Design review of the part built by this model. Coordinates are the model's own, in mm. A direction names the side the tool comes from. Give positions to 0.01 mm unless a question says otherwise; leave off trailing zeros. Write each loop counter-clockwise with the first axis right and the second up, starting at its lowest first coordinate (ties: lowest second). Pieces come first, ordered by that corner, then holes. Notation, with made-up numbers: M 56,80 L 90,80 A15 cw 90,98 Z; hole C 76.25,-8 d10. An arc over 180 degrees is marked long. One line per item, written item: value. Start each with the question number.
```python
from build123d import *

# Parameters (mm, degrees)
SKETCH_1_W            = 5.5
SKETCH_1_H            = 13
SKETCH_1_W_2          = 7
SKETCH_1_W_3          = 4
SKETCH_1_W_4          = 9
EXTRUDE_1_DEPTH       = 3
HOLE_WIZARD_M31_D     = 3.4
HOLE_WIZARD_M31_DEPTH = 10
HOLE_WIZARD_M31_TIP   = 1.021463052
FILLET_1_R            = 0.5


with BuildPart() as part:
    # Эскиз1 → Бобышка-Вытянуть1 (new body)
    with BuildSketch(Plane(origin=(0, 0, 0), x_dir=(1, 0, 0), z_dir=(0, 1, 0))):
        Polygon((-43.75, -21), (43.75, -21), (43.75, -19.5), (56.25, -19.5), (56.25, -15.5), (59.25, -15.5), (59.25, -5.5), (56.25, -5.5), (56.25, 0), (-56.25, 0), (-56.25, -5.5), (-59.25, -5.5), (-59.25, -15.5), (-56.25, -15.5), (-56.25, -19.5), (-43.75, -19.5), align=None)
        with Locations((-23.625, -9.6)):
            Rectangle(SKETCH_1_W, SKETCH_1_H, mode=Mode.SUBTRACT)
        with Locations((-33.0625, -9.6)):
            Rectangle(SKETCH_1_W, SKETCH_1_H, mode=Mode.SUBTRACT)
        with Locations((-14.1875, -9.6)):
            Rectangle(SKETCH_1_W, SKETCH_1_H, mode=Mode.SUBTRACT)
        with Locations((-4.75, -9.6)):
            Rectangle(SKETCH_1_W, SKETCH_1_H, mode=Mode.SUBTRACT)
        with Locations((16.375, -9.6)):
            Rectangle(SKETCH_1_W_2, SKETCH_1_H, mode=Mode.SUBTRACT)
        with Locations((5.4375, -9.6)):
            Rectangle(SKETCH_1_W_2, SKETCH_1_H, mode=Mode.SUBTRACT)
        with Locations((27.3125, -9.6)):
            Rectangle(SKETCH_1_W_2, SKETCH_1_H, mode=Mode.SUBTRACT)
        with Locations((-41.75, -9.6)):
            Rectangle(SKETCH_1_W_3, SKETCH_1_H, mode=Mode.SUBTRACT)
        with Locations((39.25, -9.6)):
            Rectangle(SKETCH_1_W_4, SKETCH_1_H, mode=Mode.SUBTRACT)
    extrude(amount=EXTRUDE_1_DEPTH)

    # Отверстие с зазором M31
    with Locations(Plane(origin=(0, 3, 0), x_dir=(1, 0, 0), z_dir=(0, 1, 0))):
        with Locations((50, -9.6), (-50, -9.6)):
            Hole(HOLE_WIZARD_M31_D / 2, depth=HOLE_WIZARD_M31_DEPTH)
            with Locations((0, 0, -(HOLE_WIZARD_M31_DEPTH + HOLE_WIZARD_M31_TIP / 2))):  # 118° drill point
                Cone(0, HOLE_WIZARD_M31_D / 2, HOLE_WIZARD_M31_TIP, mode=Mode.SUBTRACT)

    # Скругление1
    fillet_1_edges = [part.edges().sort_by_distance(p)[0] for p in [
        (-56.25, 1.5, 19.5),
        (-59.25, 1.5, 15.5),
        (-59.25, 1.5, 5.5),
        (-56.25, 1.5, 0),
        (56.25, 1.5, 0),
        (59.25, 1.5, 5.5),
        (59.25, 1.5, 15.5),
        (56.25, 1.5, 19.5),
    ]]
    fillet(fillet_1_edges, radius=FILLET_1_R)


solid = part.part
```
Q1. Take a section at C-C, the plane y = 2.3. State how many separate pieces and enclosed holes the cut face has, then the cut area to 3 significant figures.
Q2. Machinability: for faces 4 (the face through (-50, 1, 19.5)), 5 (the face through (-11.438, 1, 10)), which of the approach directions +Z, -Z, +X, -X, +Y, -Y give a long, thin tool a straight path to every point of the face, cutting with its end or side? Answer none if there is none.
Q3. The part is to be moulded in two halves that separate along Z. For faces 1 (the face through (-56.25, 1, 17)), 2 (the face through (34.75, 1, 10)), 3 (the face through (50, 1, 19.5)), say which applies: pulls with the +Z half, pulls with the -Z half, needs draft (parallel to the pull), parting line crosses it, or undercut.
Q4. Take a section at D-D, the plane z = 17.5. Give the boundary of the cut face in (x, y), then the cut area to 4 significant figures.
Q5. Take a section at B-B, the plane x = -50. Give the boundary of the cut face in (y, z), then the cut area to 3 significant figures.
Q6. Take a section at A-A, the plane x = 29.5. Give the boundary of the cut face in (y, z).
Q7. Wall thickness on line 1 (Z direction, x = -33, y = 0.75); line 2 (Z direction, x = 50, y = 1.1); line 3 (X direction, y = 0.1, z = 1.5): over which ranges is each line inside the solid? List them lowest first. Write a range as from..to.
Q8. For P1, Ø1.2, axis at x = -58, y = 1, coming from the -Z side; P2, Ø5, axis at x = 30.5, z = 9, coming from the -Y side; P3, Ø1.6, axis at y = 2, z = 20, coming from the -X side, all flat-tipped, find the tip position at first contact; note any pin that passes through.
Results list:
1. separate pieces: 1
1. enclosed holes: 11
1. area: 1,640 mm^2
2. face 4: +Z, -X, +Y, -Y
2. face 5: +Y, -Y
3. face 1: needs draft
3. face 2: undercut
3. face 3: pulls with the +Z half
4. outline: M -56.25,0 L 56.25,0 L 56.25,3 L -56.25,3 Z
4. area: 337.5 mm^2
5. outline: M 0,0 L 3,0 L 3,7.9 L 0,7.9 Z; M 0,11.3 L 3,11.3 L 3,19.5 L 0,19.5 Z
5. area: 48.3 mm^2
6. outline: M 0,0 L 3,0 L 3,3.1 L 0,3.1 Z; M 0,16.1 L 3,16.1 L 3,21 L 0,21 Z
7. line 1: z = 0..3.1, 16.1..21
7. line 2: z = 0..7.9, 11.3..19.5
7. line 3: x = -56.25..56.25
8. P1: stops at z = 5.5
8. P2: stops at y = 0
8. P3: stops at x = -56.21
